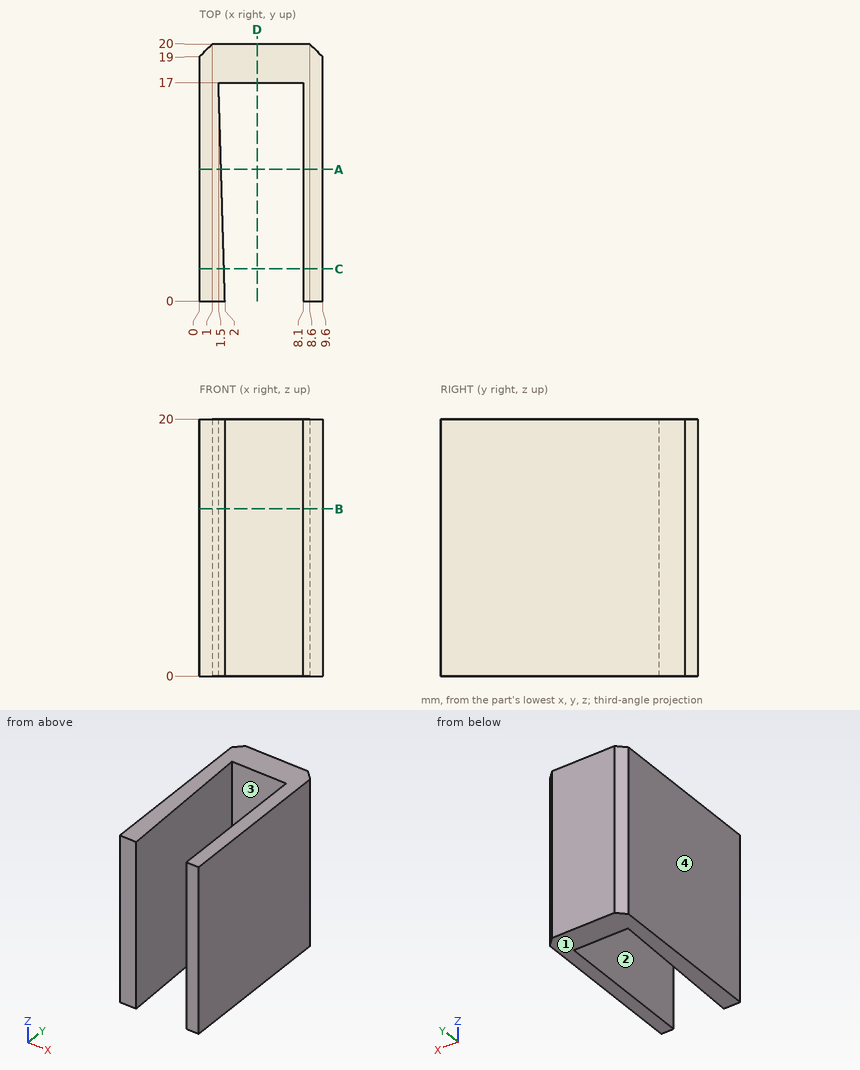
Input: dimensioned drawing with shaded views. Units: mm. Origin: part minimum x, y, z. Coordinates: 2 decimals unless noted, no trailing zeros. Loops run counter-clockwise (first coordinate to the right, second up) from the corner with the lowest first, then second, coordinate; pieces in that order, holes last. Notation, with made-up numbers: (12, 31.25) -> (63, 31.25) arc R10 ccw to (63, 43.25) -> close; hole circle Ø4 at (-26, 7.5). An arc over 180 degrees is marked (long way). Use a Markdown table: item, result. Add a question column.
(1) Section query D-D, the plane x = 4.5. Return loops of the section in (y, z).
(2) Pin query (flat end, axial travel): pin 1 Ø2 at (x, z) = (5, 11) entering from -Y; pin 2 Ø2 at (x, y) = (6.5, 3.5) entering from +Z. Return the tip coordinate at first contact, or that it passes through.
(3) Line query: line 1 along Y through (x, z) = (5.75, 17.5); line 2 along X through (y, z) = (4.5, 14.75); line 3 along X through (y, z) = (6.75, 8.5). Output: solid intervals per line, ascending.
(4) Section query B-B, the plane z = 13. Return loops of the section in (x, y).
(5) Section query A-A, the plane y = 10.25. Return loops of the section in (x, z).
(6) Mould query, pull axis X, two halves, no side actions, for the marked faces 1, 2, 3 and 4. Classes: pulls with the +X half, pulls with the -X half, needs draft (parallel to the pull), parting line crosses it, or undercut.
(7) Section query C-C, the plane y = 2.5. Return loops of the section in (x, z), plus the area to 3 significant figures.
Answer:
| question | item | result |
|---|---|---|
| 1 | outline | (17, 0) -> (20, 0) -> (20, 20) -> (17, 20) -> close |
| 2 | pin 1 | stops at y = 17 |
| 2 | pin 2 | passes through |
| 3 | line 1 | y = 17 to 20 |
| 3 | line 2 | x = 0 to 1.87, 8.1 to 9.6 |
| 3 | line 3 | x = 0 to 1.8, 8.1 to 9.6 |
| 4 | outline | (0, 0) -> (2, 0) -> (1.5, 17) -> (8.1, 17) -> (8.1, 0) -> (9.6, 0) -> (9.6, 19) -> (8.6, 20) -> (1, 20) -> (0, 19) -> close |
| 5 | outline | (0, 0) -> (1.7, 0) -> (1.7, 20) -> (0, 20) -> close; (8.1, 0) -> (9.6, 0) -> (9.6, 20) -> (8.1, 20) -> close |
| 6 | face 1 | needs draft |
| 6 | face 2 | undercut |
| 6 | face 3 | undercut |
| 6 | face 4 | pulls with the -X half |
| 7 | outline | (0, 0) -> (1.93, 0) -> (1.93, 20) -> (0, 20) -> close; (8.1, 0) -> (9.6, 0) -> (9.6, 20) -> (8.1, 20) -> close |
| 7 | area | 68.5 mm^2 |
